Part model, mm, in its own coordinate system. A direction names the side the tool comes from. Give positions to 0.01 mm unless a question says otherwise; leave off trailing zeros. Order: outer loops, then holes, each group sorted by start corner. A loop starts at its lowest first (then second) coordinate and runs counter-clockwise, first axis right, second up.
1. Which spindle directions (+Z, -Z, +X, -X, +Y, -Y) get a long thin tool onto all of the face, cutting with end or side? Do faces 1 (the conical face through (-2.67, 12.026, 6.961)), 2 (the conical face through (0.433, 3.294, -137.486)), 3 (the flat face through (0, 0, 6.35)). Say none if no direction does.
2. Slice it at D-D on z = -120. List the corners of the cut face in (x, y) (3 decimals), and give its area (3 significant figures).
3. Drop flat-ended pins along their axis: pin 1 Ø1.5 at (x, y) = (3.5, 4) entering from +Z; pin 2 Ø3 at (y, z) = (1, -74) entering from -X (3 decimals); pin 3 Ø3 at (x, z) = (5.5, -154.5) entering from +Y. Give the stop position or say it passes through.
4. Probe line 1 (Z direction, x = -7, y = 3.5); line 2 (Z direction, x = -0.25, y = 1); line 3 (Y direction, x = 2, z = -167). List the from-to ranges inside material, lowest first.
5. Slice it at C-C on z = -164.5. List the corners of the cut face in (x, y).
6. Slice it at A-A on x = 0. List the corners of the cut face in (y, z) (3 decimals).
7. Mould opens along Y. For faces 4 (the flat face through (0, 0, -177.8)), 5 (the cylindrical face through (-4.394, 3.369, -158.483)), 6 (the conical face through (10.49, -3.3, 6.63)) say: +Y half, -Y half, draft (parallel to the pull), parting line (faces both ways), or undercut.
from build123d import *

# Parameters (mm, degrees)
F2_R     = 3.81
F3_R     = 3.175
F4_DEPTH = 139.7
F5_R     = 5.5372
F6_DEPTH = 38.1


with BuildPart() as f1:
    # F0 (on Front) → F1 (revolve)
    with BuildSketch(Plane.XZ):
        Polygon((0, 6.35), (0, 0), (11.811, 0), (12.7, 12.192), (12.446, 12.192), (10.922, 6.35), align=None)
    revolve(axis=Axis((0, 0, 3.175), (0, 0, -1)))

    # F2
    f2_edges = [f1.edges().sort_by_distance(p)[0] for p in [
        (-11.811, 0, 0),
    ]]
    fillet(f2_edges, radius=F2_R)

    # F3 (on face) → F4 (join)
    with BuildSketch(Plane(origin=(0, 0, 0), x_dir=(1, 0, 0), z_dir=(0, 0, -1))):
        Circle(F3_R)
    extrude(amount=F4_DEPTH)

    # F5 (on face) → F6 (join)
    with BuildSketch(Plane(origin=(0, 0, -139.7), x_dir=(1, 0, 0), z_dir=(0, 0, -1))):
        Circle(F5_R)
    extrude(amount=F6_DEPTH)

    # F7 (on Front) → F8 (revolve)
    with BuildSketch(Plane.XZ):
        Polygon((-5.5372, -139.7), (0, -139.7), (0, -134.1628), align=None)
    revolve(axis=Axis((0, 0, -136.9314), (0, 0, -1)))


solid = f1.part
Data:
1. face 1: -Z
1. face 2: none
1. face 3: +Z
2. outline: circle Ø6.35 at (0, 0)
2. area: 31.7 mm2
3. pin 1: stops at z = 6.35
3. pin 2: stops at x = -3.175
3. pin 3: stops at y = 3.83
4. line 1: z = 0 to 6.35
4. line 2: z = -177.8 to 6.35
4. line 3: y = -5.16 to 5.16
5. outline: circle Ø11.07 at (0, 0)
6. outline: (-12.7, 12.192) - (-12.069, 3.533) arc R3.81 ccw to (-8.269, 0) - (-3.175, 0) - (-3.175, -137.338) - (-5.537, -139.7) - (-5.537, -177.8) - (5.537, -177.8) - (5.537, -139.7) - (3.175, -137.338) - (3.175, 0) - (8.269, 0) arc R3.81 ccw to (12.069, 3.533) - (12.7, 12.192) - (12.446, 12.192) - (10.922, 6.35) - (-10.922, 6.35) - (-12.446, 12.192) - close
7. face 4: draft
7. face 5: parting line
7. face 6: undercut
